Source: CAD feature listing. Evaluate the final solid. Frame: model axes, mm. Face numbers are marked on the shaded views. Round coordinates to 2 decimals unless told otherwise and drop trailing zeros. Order: outer loops, then holes, each group sorted by start corner. A loop starts at its lowest first (then second) coordinate and runs counter-clockwise, first axis right, second up. Notation, with made-up numbers: M 19.25,75.25 L 58.25,75.25 A21 ccw 58.25,80.25 Z; hole C 41,52 d10. An arc over 180 degrees is marked long. Use one line per item in the form item = value. Start each with the question number.
Q1. Contact query for flat-ended pins moving along their axis: pin 1 (1 mm diameter, centred on x = -69, z = 3, fed in from +Y); pin 2 (0.5 mm diameter, centred on y = 2.5, z = 8.5, fed in from -X) (3 decimals). Output: stop coordinate, or through.
Q2. Section C-C (x = -74.5). Return the cut outline in (y, z) (3 decimals), plus the area to 3 significant figures.
Q3. Pull-direction query (Z, two-part tool) for the marked faces 1 and 2; classes: pulls with the +Z half, pulls with the -Z half, needs draft (parallel to the pull), parting line crosses it, or undercut.
Q4. Section A-A (x = -68). Return the cut outline in (y, z) (3 decimals).
Q5. Section B-B (z = 16). Return the cut outline in (x, y) (3 decimals).
Q6. Material intervals for probe 1 along X at (y, z) = (2.1, 8) (3 decimals); probe 2 along Z at (x, y) = (-71.5, 0.45) (3 decimals); probe 3 along Z at (x, y) = (-28, 2.35), sorted ascending.
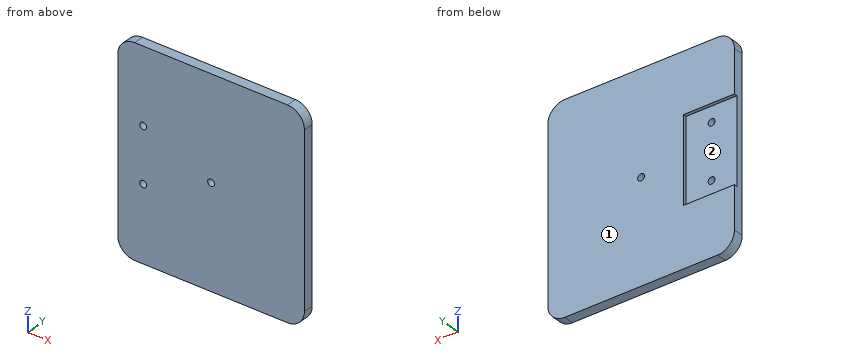
from build123d import *

# Parameters (mm, degrees)
SKETCH2_W           = 55
SKETCH2_H           = 60
BOSS_EXTRUDE1_DEPTH = 3
SKETCH3_W           = 15
SKETCH3_H           = 25
CUT_EXTRUDE1_DEPTH  = 1
SKETCH4_R           = 1
CUT_EXTRUDE3_DEPTH  = 5
FILLET1_R           = 5
SKETCH5_R           = 1
CUT_EXTRUDE4_DEPTH  = 5


with BuildPart() as part:
    # Sketch2 → Boss-Extrude1 (new body)
    with BuildSketch(Plane(origin=(0, 0, 0), x_dir=(1, 0, 0), z_dir=(0, 1, 0))):
        with Locations((-50.625, -5.625)):
            Rectangle(SKETCH2_W, SKETCH2_H)
    extrude(amount=BOSS_EXTRUDE1_DEPTH)

    # Sketch3 → Cut-Extrude1 (cut)
    with BuildSketch(Plane(origin=(0, 3, 0), x_dir=(1, 0, 0), z_dir=(0, 1, 0))):
        with Locations((-70.625, -5.625)):
            Rectangle(SKETCH3_W, SKETCH3_H)
    extrude(amount=-CUT_EXTRUDE1_DEPTH, mode=Mode.SUBTRACT)

    # Sketch4 → Cut-Extrude3 (cut)
    with BuildSketch(Plane(origin=(0, 3, 0), x_dir=(1, 0, 0), z_dir=(0, 1, 0))):
        with Locations(Location((-70.625, 2.375, 0), (0, 0, 270))):
            Circle(SKETCH4_R)
        with Locations(Location((-70.625, -13.625, 0), (0, 0, 270))):
            Circle(SKETCH4_R)
    extrude(amount=-CUT_EXTRUDE3_DEPTH, mode=Mode.SUBTRACT)

    # Fillet1
    fillet1_edges = [part.edges().sort_by_distance(p)[0] for p in [
        (-78.125, 1.5, -24.375),
        (-23.125, 1.5, -24.375),
        (-23.125, 1.5, 35.625),
        (-78.125, 1.5, 35.625),
    ]]
    fillet(fillet1_edges, radius=FILLET1_R)

    # Sketch5 → Cut-Extrude4 (cut)
    with BuildSketch(Plane(origin=(0, 3, 0), x_dir=(1, 0, 0), z_dir=(0, 1, 0))):
        with Locations(Location((-50.625, -5.625, 0), (0, 0, 270))):
            Circle(SKETCH5_R)
    extrude(amount=-CUT_EXTRUDE4_DEPTH, mode=Mode.SUBTRACT)


solid = part.part
Results list:
q1.pin_1 = 2
q1.pin_2 = -63.125
q2.outline = M 0,-24.182 L 3,-24.182 L 3,-6.875 L 2,-6.875 L 2,18.125 L 3,18.125 L 3,35.432 L 0,35.432 Z
q2.area = 154 mm2
q3.face_1 = needs draft
q3.face_2 = undercut
q4.outline = M 0,-24.375 L 3,-24.375 L 3,-6.875 L 2,-6.875 L 2,18.125 L 3,18.125 L 3,35.625 L 0,35.625 Z
q5.outline = M -78.125,0 L -23.125,0 L -23.125,3 L -63.125,3 L -63.125,2 L -78.125,2 Z
q6.probe_1 = -63.125 to -23.125
q6.probe_2 = -24.375 to -2.859, -1.891 to 13.141, 14.109 to 35.625
q6.probe_3 = -24.37 to 35.62
